Design review of the part built by this model. Coordinates are the model's own, in mm. Face numbers are marked on the shaded views. A direction names the side the tool comes from. Round coordinates to 2 decimals unless told otherwise and drop trailing zeros. Order: outer loops, then holes, each group sorted by start corner. A loop starts at its lowest first (then second) coordinate and runs counter-clockwise, first axis right, second up. Notation, with made-up numbers: (-28.75, 18.25) - (21.25, 18.25) arc R31 cw to (21.25, 48.25) - close; hole circle Ø10 at (68.5, 63.5). An arc over 180 degrees is marked (long way). Use CSV: the item, a comma, the result in double quotes.
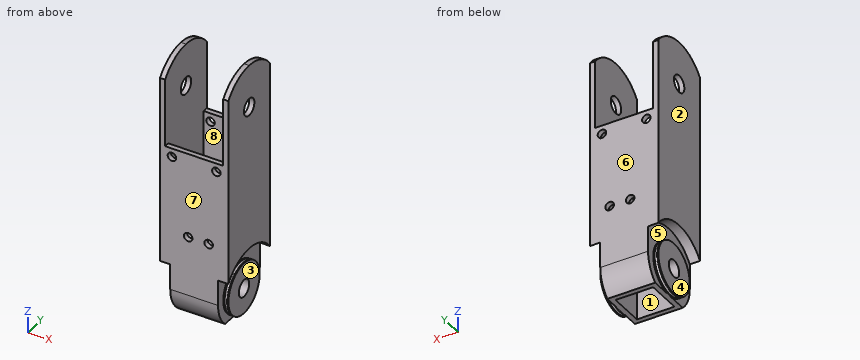
from build123d import *

# Parameters (mm, degrees)
CROQUIS1_W              = 40
CROQUIS1_H              = 40
SALIENTE_EXTRUIR1_DEPTH = 150
CROQUIS2_W              = 34
CROQUIS2_H              = 40
CORTAR_EXTRUIR1_DEPTH   = 50
CORTAR_EXTRUIR5_DEPTH   = 157.524758425
CROQUIS4_R              = 5
CORTAR_EXTRUIR6_DEPTH   = 157.524758425
CORTAR_EXTRUIR10_DEPTH  = 157.524758425
CROQUIS5_R              = 5
CORTAR_EXTRUIR7_DEPTH   = 157.524758425
CROQUIS6_R              = 5
CORTAR_EXTRUIR8_DEPTH   = 6
CORTAR_EXTRUIR11_START  = -6
CROQUIS9_R              = 5
CORTAR_EXTRUIR11_DEPTH  = 6
SALIENTE_EXTRUIR2_START = 3
CROQUIS10_R             = 15
CROQUIS10_R_2           = 5
SALIENTE_EXTRUIR2_DEPTH = 3
CROQUIS11_R             = 15
CROQUIS11_R_2           = 5
SALIENTE_EXTRUIR3_DEPTH = 3
CROQUIS12_R             = 0.75
CROQUIS13_R             = 2.5
CORTAR_EXTRUIR12_DEPTH  = 157.524758425
CROQUIS15_W             = 22
CROQUIS15_H             = 20.45751311
CORTAR_EXTRUIR14_DEPTH  = 95
CROQUIS17_W             = 34
CROQUIS17_H             = 34
CORTAR_EXTRUIR15_DEPTH  = 55
CROQUIS18_R             = 2.5
CORTAR_EXTRUIR16_DEPTH  = 157.524758425


with BuildPart() as part:
    # Croquis1 → Saliente-Extruir1 (new body)
    with BuildSketch(Plane.XY):
        Rectangle(CROQUIS1_W, CROQUIS1_H)
    extrude(amount=SALIENTE_EXTRUIR1_DEPTH)

    # Croquis2 → Cortar-Extruir1 (cut)
    with BuildSketch(Plane.XY.offset(150)):
        Rectangle(CROQUIS2_W, CROQUIS2_H)
    extrude(amount=-CORTAR_EXTRUIR1_DEPTH, mode=Mode.SUBTRACT)

    # Croquis3 → Cortar-Extruir5 (cut, through all)
    with BuildSketch(Plane(origin=(20, 0, 0), x_dir=(0, 0, -1), z_dir=(1, 0, 0))):
        with BuildLine():
            ThreePointArc((-140, -20), (-147.360679775, -11.180339887), (-150, 0))
            Line((-150, 0), (-150, -20))
            Line((-150, -20), (-140, -20))
        make_face()
        with BuildLine():
            Line((-140, 20), (-150, 20))
            Line((-150, 20), (-150, 0))
            ThreePointArc((-150, 0), (-147.360679775, 11.180339887), (-140, 20))
        make_face()
    extrude(amount=-CORTAR_EXTRUIR5_DEPTH, mode=Mode.SUBTRACT)

    # Croquis4 → Cortar-Extruir6 (cut, through all)
    with BuildSketch(Plane(origin=(20, 0, 0), x_dir=(0, 0, -1), z_dir=(1, 0, 0))):
        with Locations((-125, 0)):
            Circle(CROQUIS4_R)
    extrude(amount=-CORTAR_EXTRUIR6_DEPTH, mode=Mode.SUBTRACT)

    # Croquis8 → Cortar-Extruir10 (cut, through all)
    with BuildSketch(Plane(origin=(20, 0, 0), x_dir=(0, 0, -1), z_dir=(1, 0, 0))):
        with BuildLine():
            Line((0, 20), (-15, 20))
            ThreePointArc((-15, 20), (-6.771243445, 18.228756555), (0, 13.228756555))
            Line((0, 13.228756555), (0, 20))
        make_face()
        with BuildLine():
            Line((0, -20), (0, -13.228756555))
            ThreePointArc((0, -13.228756555), (-6.771243445, -18.228756555), (-15, -20))
            Line((-15, -20), (0, -20))
        make_face()
    extrude(amount=-CORTAR_EXTRUIR10_DEPTH, mode=Mode.SUBTRACT)

    # Croquis5 → Cortar-Extruir7 (cut, through all)
    with BuildSketch(Plane(origin=(20, 0, 0), x_dir=(0, 0, -1), z_dir=(1, 0, 0))):
        with Locations((-15, 0)):
            Circle(CROQUIS5_R)
    extrude(amount=-CORTAR_EXTRUIR7_DEPTH, mode=Mode.SUBTRACT)

    # Croquis6 → Cortar-Extruir8 (cut)
    with BuildSketch(Plane(origin=(20, 0, 0), x_dir=(0, 0, -1), z_dir=(1, 0, 0))):
        with BuildLine():
            ThreePointArc((-30, 20), (-40, 0), (-30, -20))
            Line((-30, -20), (-15, -20))
            ThreePointArc((-15, -20), (-6.771243445, -18.228756555), (0, -13.228756555))
            Line((0, -13.228756555), (0, 13.228756555))
            ThreePointArc((0, 13.228756555), (-6.771243445, 18.228756555), (-15, 20))
            Line((-15, 20), (-30, 20))
        make_face()
        with Locations((-15, 0)):
            Circle(CROQUIS6_R, mode=Mode.SUBTRACT)
    extrude(amount=-CORTAR_EXTRUIR8_DEPTH, mode=Mode.SUBTRACT)

    # Croquis9 → Cortar-Extruir11 (cut)
    with BuildSketch(Plane.ZY.offset(20).offset(CORTAR_EXTRUIR11_START)):
        with BuildLine():
            ThreePointArc((30, -20), (40, 0), (30, 20))
            Line((30, 20), (15, 20))
            ThreePointArc((15, 20), (6.771243445, 18.228756555), (0, 13.228756555))
            Line((0, 13.228756555), (0, -13.228756555))
            ThreePointArc((0, -13.228756555), (6.771243445, -18.228756555), (15, -20))
            Line((15, -20), (30, -20))
        make_face()
        with Locations(Location((15, 0, 0), (0, 0, 180))):
            Circle(CROQUIS9_R, mode=Mode.SUBTRACT)
    extrude(amount=CORTAR_EXTRUIR11_DEPTH, mode=Mode.SUBTRACT)

    # Croquis10 → Saliente-Extruir2 (add)
    with BuildSketch(Plane(origin=(14, 0, 0), x_dir=(0, 0, -1), z_dir=(1, 0, 0)).offset(SALIENTE_EXTRUIR2_START)):
        with Locations((-15, 0)):
            Circle(CROQUIS10_R)
        with Locations((-15, 0)):
            Circle(CROQUIS10_R_2, mode=Mode.SUBTRACT)
    extrude(amount=-SALIENTE_EXTRUIR2_DEPTH)

    # Croquis11 → Saliente-Extruir3 (add)
    with BuildSketch(Plane.ZY.offset(14)):
        with Locations(Location((15, 0, 0), (0, 0, 180))):
            Circle(CROQUIS11_R)
        with Locations(Location((15, 0, 0), (0, 0, 180))):
            Circle(CROQUIS11_R_2, mode=Mode.SUBTRACT)
    extrude(amount=SALIENTE_EXTRUIR3_DEPTH)

    # Croquis12 → Cortar-Revolución1 (revolve, cut)
    with BuildSketch(Plane.XY.offset(15), mode=Mode.PRIVATE) as cortar_revoluci_n1_sk:
        with Locations((15.5, 15)):
            Circle(CROQUIS12_R)
        with Locations((-15.5, 15)):
            Circle(CROQUIS12_R)
    revolve(cortar_revoluci_n1_sk.sketch.rotate(Axis((-18, 0, 15), (1, 0, 0)), 270), axis=Axis((-18, 0, 15), (1, 0, 0)), mode=Mode.SUBTRACT)

    # Croquis13 → Cortar-Extruir12 (cut, through all)
    with BuildSketch(Plane.XZ.offset(20)):
        with Locations(Location((13, 95, 0), (0, 0, 270))):
            Circle(CROQUIS13_R)
        with Locations(Location((-13, 95, 0), (0, 0, 270))):
            Circle(CROQUIS13_R)
    extrude(amount=-CORTAR_EXTRUIR12_DEPTH, mode=Mode.SUBTRACT)

    # Croquis15 → Cortar-Extruir14 (cut)
    with BuildSketch(Plane(origin=(0, 0, 0), x_dir=(-1, 0, 0), z_dir=(0, 0, -1))):
        Rectangle(CROQUIS15_W, CROQUIS15_H)
    extrude(amount=-CORTAR_EXTRUIR14_DEPTH, mode=Mode.SUBTRACT)

    # Croquis17 → Cortar-Extruir15 (cut)
    with BuildSketch(Plane.XY.offset(100)):
        Rectangle(CROQUIS17_W, CROQUIS17_H)
    extrude(amount=-CORTAR_EXTRUIR15_DEPTH, mode=Mode.SUBTRACT)

    # Croquis18 → Cortar-Extruir16 (cut, through all)
    with BuildSketch(Plane(origin=(0, 20, 0), x_dir=(1, 0, 0), z_dir=(0, 1, 0))):
        with Locations(Location((8.5, -50, 0), (0, 0, 270))):
            Circle(CROQUIS18_R)
        with Locations(Location((-3.5, -50, 0), (0, 0, 270))):
            Circle(CROQUIS18_R)
    extrude(amount=-CORTAR_EXTRUIR16_DEPTH, mode=Mode.SUBTRACT)


solid = part.part
1) Insertion check: pin 1 Ø2 at (x, y) = (8.5, -13.5) entering from +Z; pin 2 Ø3 at (x, z) = (-3.5, 50) entering from -Y; pin 3 Ø8 at (x, y) = (1, -13.5) entering from +Z; pin 4 Ø16 at (y, z) = (0, 15) entering from +X. Each pin has a flat end and moves straight along its axis. Give the tip position at first contact, or say it passes through.
Data:
pin 1,"stops at z = 45"
pin 2,"passes through"
pin 3,"stops at z = 100"
pin 4,"stops at x = 17"
2) For the marked faces 4, 5, 6, 7 and 8, list the 3-axis set-ups (+Z, -Z, +X, -X, +Y, -Y) from which the entire face can be reached by the end or side of a thin tool; tool diameter is ignored.
Data:
face 4,"-Z, -X, +Y, -Y"
face 5,"-X"
face 6,"+Z, -Z, +X, -X, +Y"
face 7,"+Z, -Z, +X, -X, -Y"
face 8,"+Z"
3) To check wall thickness, follow L1, parallel to X at y = -17.95, z = 50; L2, parallel to X at y = 9.5, z = 105.5; L3, parallel to X at y = 0, z = 42.5. State the ranges of each line that lie inside material, in increasing order. Write a range as from..to.
Data:
L1,"x = -20..-6, -1..6, 11..20"
L2,"x = -20..-17, 17..20"
L3,"x = -20..-11, 11..20"
4) We need section A-A (z = 95). Give the boundary of the cut face in (x, y).
Data:
outline,"(-20, -20) - (-15.5, -20) - (-15.5, -17) - (-17, -17) - (-17, 17) - (-15.5, 17) - (-15.5, 20) - (-20, 20) - close; (-10.5, -20) - (10.5, -20) - (10.5, -17) - (-10.5, -17) - close; (-10.5, 17) - (10.5, 17) - (10.5, 20) - (-10.5, 20) - close; (15.5, -20) - (20, -20) - (20, 20) - (15.5, 20) - (15.5, 17) - (17, 17) - (17, -17) - (15.5, -17) - close"
5) The part is to be moulded in two halves that separate along X. For the marked faces 1, 2 and 3, say which applies: +X half, -X half, draft (parallel to the pull), parting line (faces both ways), or undercut.
Data:
face 1,"undercut"
face 2,"-X half"
face 3,"+X half"
6) We need section C-C (z = 59). Give the boundary of the cut face in (x, y), then the cut area to 3 significant figures.
Data:
outline,"(-20, -20) - (20, -20) - (20, 20) - (-20, 20) - close; hole (-17, -17) - (17, -17) - (17, 17) - (-17, 17) - close"
area,"444 mm2"
7) We need section B-B (x = -7.5). Give the boundary of the cut face in (y, z).
Data:
outline,"(-20, 15) arc R20 ccw to (-13.23, 0) - (-10.23, 0) - (-10.23, 45) - (-17, 45) - (-17, 100) - (-20, 100) - close; (10.23, 0) - (13.23, 0) arc R20 ccw to (20, 15) - (20, 100) - (17, 100) - (17, 45) - (10.23, 45) - close"
